Input: part model. Units: mm. Frame: model coordinates. Coordinates: 2 decimals unless noted, no trailing zeros. Loops run counter-clockwise (first coordinate to the right, second up) from the corner with the lowest first, then second, coordinate; pieces in that order, holes last.
Item 1: Section B-B on z = -46.5. Return loops of the section in (x, y).
Item 2: Section A-A on x = -44. Return loops of the section in (y, z).
Item 3: Contact query for flat-ended pins moving along their axis: P1, Ø2.5, axis at x = -29.59, z = -51.25, coming from the -Y side; P2, Ø2, axis at y = 3.5, z = -62, coming from the +X side; P3, Ø1.5, axis at x = 15.5, y = 0.5, coming from the +Z side; P4, Ø1, axis at y = 2, z = 19, coming from the -X side. Output: stop coordinate, or through.
Item 4: Section C-C on y = 2.9. Give the number of separate pieces and of enclosed holes in the cut face, and give its area (3 significant figures).
Item 5: Ray query, line 1 along X through (y, z) = (1.2, 0); line 2 along Z through (x, y) = (-70, 2.3); line 3 along X through (y, z) = (0.8, -30). Return the intervals inside material, ascending.
```python
from build123d import *

# Parameters (mm, degrees)
SKETCH1_R           = 79
SKETCH1_R_2         = 1
SKETCH1_R_3         = 49.3
SKETCH1_R_4         = 1.6
BOSS_EXTRUDE1_DEPTH = 4


with BuildPart() as part:
    # Sketch1 → Boss-Extrude1 (new body)
    with BuildSketch(Plane(origin=(0, 0, 0), x_dir=(1, 0, 0), z_dir=(0, 1, 0))):
        with Locations(Location((0, 0, 0), (0, 0, 270))):
            Circle(SKETCH1_R)
        with Locations(Location((0, 59.18, 0), (0, 0, 270))):
            Circle(SKETCH1_R_2, mode=Mode.SUBTRACT)
        with Locations(Location((29.59, 51.251383396, 0), (0, 0, 270))):
            Circle(SKETCH1_R_2, mode=Mode.SUBTRACT)
        with Locations(Location((51.251383396, 29.59, 0), (0, 0, 270))):
            Circle(SKETCH1_R_2, mode=Mode.SUBTRACT)
        with Locations(Location((59.18, 0, 0), (0, 0, 270))):
            Circle(SKETCH1_R_2, mode=Mode.SUBTRACT)
        with Locations(Location((51.251383396, -29.59, 0), (0, 0, 270))):
            Circle(SKETCH1_R_2, mode=Mode.SUBTRACT)
        with Locations(Location((29.59, -51.251383396, 0), (0, 0, 270))):
            Circle(SKETCH1_R_2, mode=Mode.SUBTRACT)
        with Locations(Location((0, -59.18, 0), (0, 0, 270))):
            Circle(SKETCH1_R_2, mode=Mode.SUBTRACT)
        with Locations(Location((-29.59, -51.251383396, 0), (0, 0, 270))):
            Circle(SKETCH1_R_2, mode=Mode.SUBTRACT)
        with Locations(Location((-51.251383396, -29.59, 0), (0, 0, 270))):
            Circle(SKETCH1_R_2, mode=Mode.SUBTRACT)
        with Locations(Location((-59.18, 0, 0), (0, 0, 270))):
            Circle(SKETCH1_R_2, mode=Mode.SUBTRACT)
        with Locations(Location((-51.251383396, 29.59, 0), (0, 0, 270))):
            Circle(SKETCH1_R_2, mode=Mode.SUBTRACT)
        with Locations(Location((-29.59, 51.251383396, 0), (0, 0, 270))):
            Circle(SKETCH1_R_2, mode=Mode.SUBTRACT)
        with Locations(Location((0, 0, 0), (0, 0, 270))):
            Circle(SKETCH1_R_3, mode=Mode.SUBTRACT)
        with Locations(Location((0, 70, 0), (0, 0, 270))):
            Circle(SKETCH1_R_4, mode=Mode.SUBTRACT)
        with Locations(Location((35, 60.621778265, 0), (0, 0, 270))):
            Circle(SKETCH1_R_4, mode=Mode.SUBTRACT)
        with Locations(Location((60.621778265, 35, 0), (0, 0, 270))):
            Circle(SKETCH1_R_4, mode=Mode.SUBTRACT)
        with Locations(Location((70, 0, 0), (0, 0, 270))):
            Circle(SKETCH1_R_4, mode=Mode.SUBTRACT)
        with Locations(Location((60.621778265, -35, 0), (0, 0, 270))):
            Circle(SKETCH1_R_4, mode=Mode.SUBTRACT)
        with Locations(Location((35, -60.621778265, 0), (0, 0, 270))):
            Circle(SKETCH1_R_4, mode=Mode.SUBTRACT)
        with Locations(Location((0, -70, 0), (0, 0, 270))):
            Circle(SKETCH1_R_4, mode=Mode.SUBTRACT)
        with Locations(Location((-35, -60.621778265, 0), (0, 0, 270))):
            Circle(SKETCH1_R_4, mode=Mode.SUBTRACT)
        with Locations(Location((-60.621778265, -35, 0), (0, 0, 270))):
            Circle(SKETCH1_R_4, mode=Mode.SUBTRACT)
        with Locations(Location((-70, 0, 0), (0, 0, 270))):
            Circle(SKETCH1_R_4, mode=Mode.SUBTRACT)
        with Locations(Location((-60.621778265, 35, 0), (0, 0, 270))):
            Circle(SKETCH1_R_4, mode=Mode.SUBTRACT)
        with Locations(Location((-35, 60.621778265, 0), (0, 0, 270))):
            Circle(SKETCH1_R_4, mode=Mode.SUBTRACT)
    extrude(amount=BOSS_EXTRUDE1_DEPTH)


solid = part.part
```
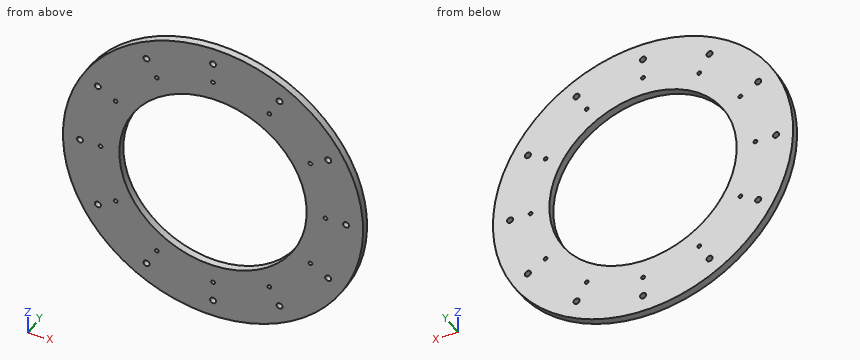
Results found:
1. outline: (-63.87, 0) - (-16.38, 0) - (-16.38, 4) - (-63.87, 4) - close; (16.38, 0) - (63.87, 0) - (63.87, 4) - (16.38, 4) - close
2. outline: (0, -65.61) - (4, -65.61) - (4, -22.24) - (0, -22.24) - close; (0, 22.24) - (4, 22.24) - (4, 65.61) - (0, 65.61) - close
3. P1: stops at y = 0
3. P2: stops at x = 50.2
3. P3: stops at z = 77.61
3. P4: stops at x = -76.8
4. separate pieces: 1
4. enclosed holes: 25
4. area: 11,800 mm2
5. line 1: x = -79 to -71.6, -68.4 to -60.18, -58.18 to -49.3, 49.3 to 58.18, 60.18 to 68.4, 71.6 to 79
5. line 2: z = -36.62 to -1.6, 1.6 to 36.62
5. line 3: x = -73.08 to -52.16, -50.34 to -39.12, 39.12 to 50.34, 52.16 to 73.08
